The figure shows three views and two pictorial views of one solid part (mm, origin at its lowest corner). Answer the questions. A direction names the side the tool comes from. Coordinates: 2 decimals unless noted, no trailing zeros. Order: outer loops, then holes, each group sorted by start corner. A loop starts at its lowest first (then second) coordinate and runs counter-clockwise, first axis right, second up. Notation, with made-up numbers: (60, 65.5) - (73, 65.5) arc R22 ccw to (73, 72.5) - close; hole circle Ø10 at (38, 87.5). An arc over 180 degrees is marked (long way). Use one line per item in the form item = value. Start each with the question number.
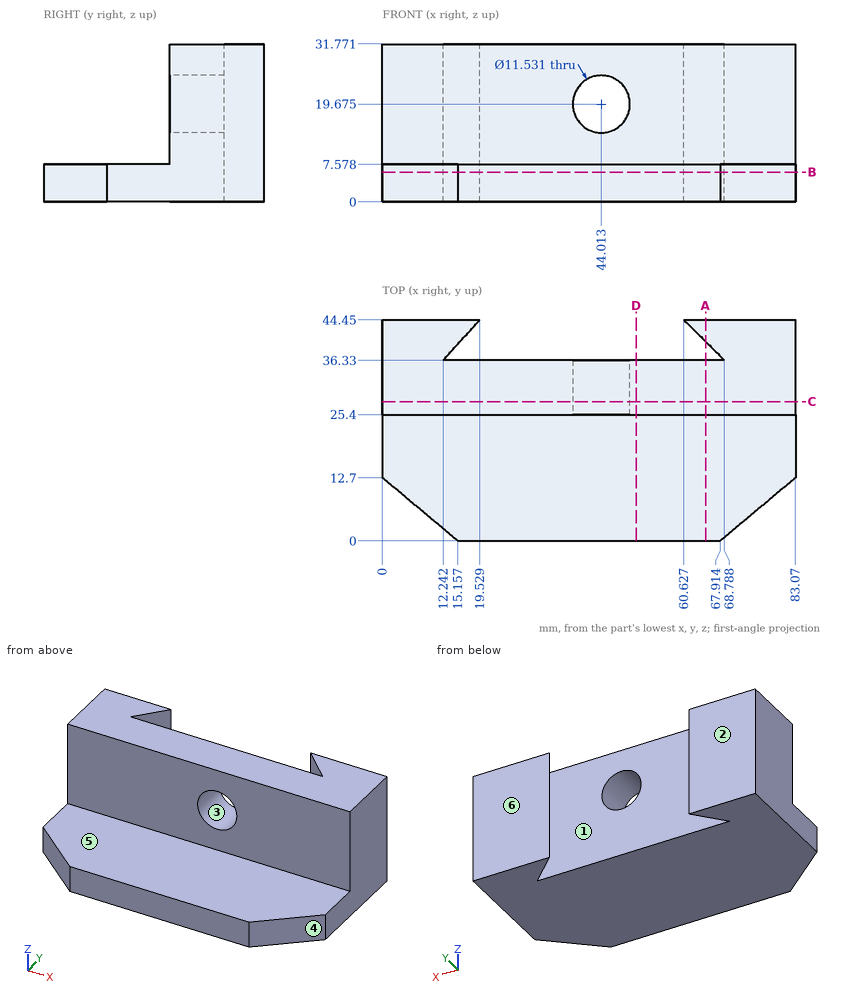
Q1. For a pull along Y with two mould halves and no side action, classify the marked faces 1, 2, 3 and 4 as +Y half, -Y half, draft (parallel to the pull), parting line (faces both ways), or undercut.
Q2. A cutting plane is placed at B-B (z = 6). Give the vertices of the cut face in (x, y).
Q3. Consider probe 1 along Y at (x, z) = (34, 8.5); probe 2 along Y at (x, z) = (27, 4); probe 3 along Z at (x, y) = (71, 3). Determine where each line is inside the solid, lowest interval first.
Q4. Given P1, Ø1.5, axis at x = 31, y = 15.5, coming from the +Z side; P2, Ø18.5, axis at x = 44.01, z = 19.67, coming from the -Y side; P3, Ø12, axis at x = 33, z = 11, coming from the -Y side; P4, Ø9.5, axis at x = 39, z = 22.5, coming from the +Y side, each flat-ended and moving along its own axis, determine where each tip first touches the part or whether it passes through.
Q5. A cutting plane is placed at C-C (y = 28). Give the vertices of the cut face in (x, z) (1 decimal).
Q6. Which of the six approach directions +Z, -Z, +X, -X, +Y, -Y give full straight-line access (tool end or side, diameter ignored) to the marked faces 5 and 6?
Q7. A cutting plane is placed at D-D (x = 51). Give the vertices of the cut face in (y, z), then the cut area to 3 significant figures.
Q8. A cutting plane is placed at A-A (x = 65). Give the vertices of the cut face in (y, z).
Result sheet:
q1.face_1 = undercut
q1.face_2 = +Y half
q1.face_3 = draft
q1.face_4 = -Y half
q2.outline = (0, 12.7) - (15.16, 0) - (67.91, 0) - (83.07, 12.7) - (83.07, 44.45) - (60.63, 44.45) - (68.79, 36.33) - (12.24, 36.33) - (19.53, 44.45) - (0, 44.45) - close
q3.probe_1 = 25.4 to 36.33
q3.probe_2 = 0 to 36.33
q3.probe_3 = 0 to 7.58
q4.P1 = 7.58
q4.P2 = 25.4
q4.P3 = 0
q4.P4 = 36.33
q5.outline = (0, 0) - (83.1, 0) - (83.1, 31.8) - (0, 31.8) - close; hole circle Ø11.5 at (44, 19.7)
q6.face_5 = +Z, +X, -X, -Y
q6.face_6 = +Z, -Z, +X, -X, +Y
q7.outline = (0, 0) - (36.33, 0) - (36.33, 31.77) - (25.4, 31.77) - (25.4, 7.58) - (0, 7.58) - close
q7.area = 540 mm^2
q8.outline = (0, 0) - (36.33, 0) - (36.33, 31.77) - (25.4, 31.77) - (25.4, 7.58) - (0, 7.58) - close; (40.1, 0) - (44.45, 0) - (44.45, 31.77) - (40.1, 31.77) - close
